Check sheet for the drawn part. Datum: minimum x, y, z corner. Units: mm. Round coordinates to 2 decimals unless told otherwise and drop trailing zeros. Write each loop counter-clockwise with the first axis right and the second up, starting at its lowest first coordinate (ties: lowest second). Pieces come first, ordered by that corner, then holes. Notation, with made-up numbers: (88.25, -9.75) - (145.25, -9.75) arc R29 cw to (145.25, 26.25) - close; hole circle Ø3 at (-34, 30.25). An arc over 180 degrees is marked (long way). Answer as a JSON object with one key per item and string values.
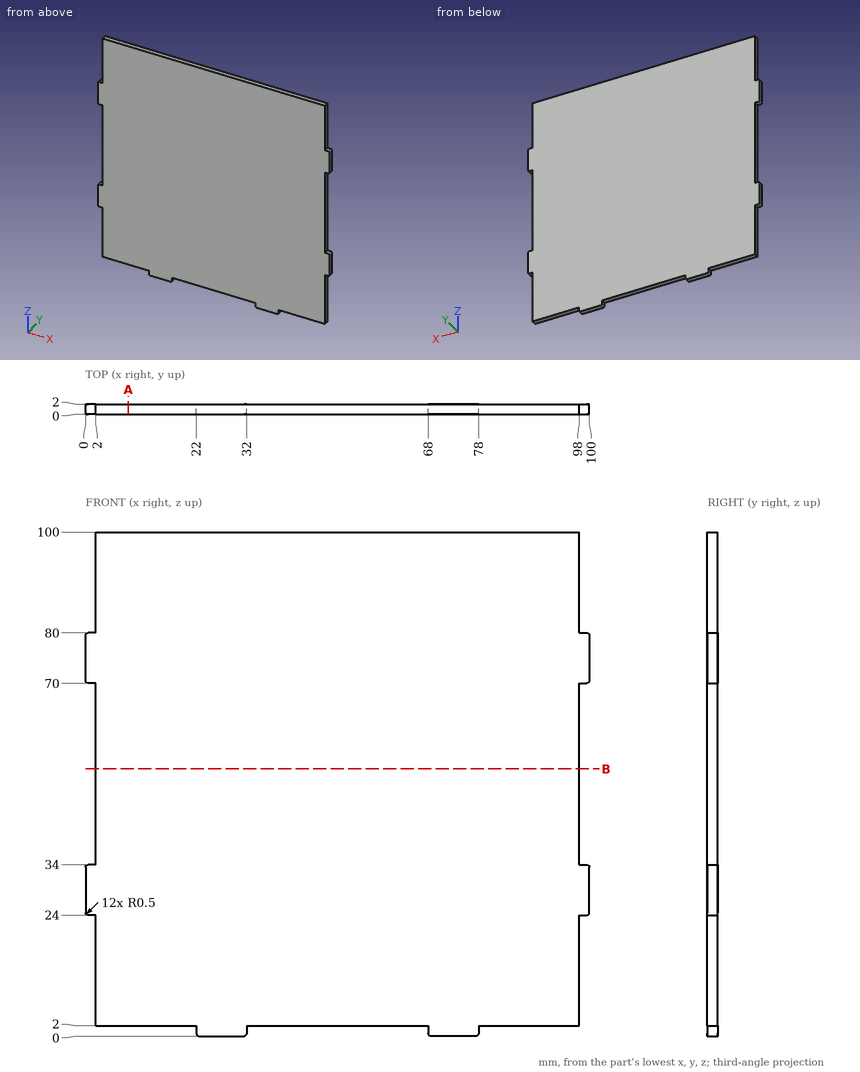
Q1. Gauge pin test, flat ends, axial feed: P1, Ø1.2, axis at x = 1.5, y = 1, coming from the -Z side; P2, Ø0.8, axis at x = 99, y = 1, coming from the +Z side; P3, Ø0.8, axis at x = 99, y = 1, coming from the -Z side. Record the tip position at first contact, or that the pin passes through.
Geometry check:
{"P1": "stops at z = 2", "P2": "stops at z = 80", "P3": "stops at z = 24"}
Q2. Material ranges on line 1 along X through (y, z) = (1.85, 14); line 2 along Z through (x, y) = (4.5, 0.55), recorded low to high. Write a range as [from, to].
Geometry check:
{"line 1": "x = [2, 98]", "line 2": "z = [2, 100]"}
Q3. Section check B-B, the plane z = 53. Record the cut outline in (x, y).
Geometry check:
{"outline": "(2, 0) - (98, 0) - (98, 2) - (2, 2) - close"}
Q4. Section check A-A, the plane x = 8.5. Record the cut outline in (y, z).
Geometry check:
{"outline": "(0, 2) - (2, 2) - (2, 100) - (0, 100) - close"}
